For this review, take the finished solid that the model builds, in its own axes (mm). A direction names the side the tool comes from. Round coordinates to 2 decimals unless told otherwise and drop trailing zeros. Order: outer loops, then holes, each group sorted by start corner. A loop starts at its lowest first (then second) coordinate and runs counter-clockwise, first axis right, second up. Notation, with made-up numbers: M 64.25,56.25 L 91.25,56.25 A22 ccw 91.25,62.25 Z; hole C 10,-1 d10. An arc over 180 degrees is marked long. Answer as a JSON object with one key per item and string values.
from build123d import *

# Parameters (mm, degrees)
SKETCH1_R           = 18.5
BOSS_EXTRUDE1_DEPTH = 22
SKETCH2_R           = 16.5
BOSS_EXTRUDE2_DEPTH = 22
SKETCH3_R           = 16.55
BOSS_EXTRUDE3_DEPTH = 1
SKETCH4_R           = 6.5
BOSS_EXTRUDE4_DEPTH = 6
SKETCH6_R           = 3
BOSS_EXTRUDE5_DEPTH = 15.5
CUT_EXTRUDE1_DEPTH  = 12
SKETCH8_R           = 1.5
CUT_EXTRUDE2_DEPTH  = 10


with BuildPart() as part:
    # Sketch1 → Boss-Extrude1 (new body)
    with BuildSketch(Plane(origin=(0, 0, 0), x_dir=(1, 0, 0), z_dir=(0, 1, 0))):
        with Locations(Location((0, 0, 0), (0, 0, 270))):
            Circle(SKETCH1_R)
    extrude(amount=BOSS_EXTRUDE1_DEPTH)

    # Sketch2 → Boss-Extrude2 (add)
    with BuildSketch(Plane.XZ):
        with Locations(Location((0, 0, 0), (0, 0, 270))):
            Circle(SKETCH2_R)
    extrude(amount=BOSS_EXTRUDE2_DEPTH)

    # Sketch3 → Boss-Extrude3 (add)
    with BuildSketch(Plane.XZ.offset(22)):
        with Locations(Location((0, 0, 0), (0, 0, 270))):
            Circle(SKETCH3_R)
    extrude(amount=BOSS_EXTRUDE3_DEPTH)

    # Sketch4 → Boss-Extrude4 (add)
    with BuildSketch(Plane(origin=(0, 22, 0), x_dir=(1, 0, 0), z_dir=(0, 1, 0))):
        with Locations(Location((0, 7, 0), (0, 0, 270))):
            Circle(SKETCH4_R)
    extrude(amount=BOSS_EXTRUDE4_DEPTH)

    # Sketch6 → Boss-Extrude5 (add)
    with BuildSketch(Plane(origin=(0, 28, 0), x_dir=(1, 0, 0), z_dir=(0, 1, 0))):
        with Locations(Location((0, 7, 0), (0, 0, 270))):
            Circle(SKETCH6_R)
    extrude(amount=BOSS_EXTRUDE5_DEPTH)

    # Sketch7 → Cut-Extrude1 (cut)
    with BuildSketch(Plane(origin=(0, 43.5, 0), x_dir=(1, 0, 0), z_dir=(0, 1, 0))):
        Polygon((-2.084617871, 9.15739851), (2.084617871, 9.15739851), (2.280696351, 9.15739851), (2.280696351, 10.992904137), (-3.0808507, 10.992904137), (-3.0808507, 9.15739851), align=None)
    extrude(amount=-CUT_EXTRUDE1_DEPTH, mode=Mode.SUBTRACT)

    # Sketch8 → Cut-Extrude2 (cut)
    with BuildSketch(Plane(origin=(0, 22, 0), x_dir=(1, 0, 0), z_dir=(0, 1, 0))):
        with Locations(Location((15.5, 0, 0), (0, 0, 270))):
            Circle(SKETCH8_R)
        with Locations(Location((7.75, -13.423393759, 0), (0, 0, 270))):
            Circle(SKETCH8_R)
        with Locations(Location((-7.75, -13.423393759, 0), (0, 0, 270))):
            Circle(SKETCH8_R)
        with Locations(Location((-15.5, 0, 0), (0, 0, 270))):
            Circle(SKETCH8_R)
        with Locations(Location((-7.75, 13.423393759, 0), (0, 0, 270))):
            Circle(SKETCH8_R)
        with Locations(Location((7.75, 13.423393759, 0), (0, 0, 270))):
            Circle(SKETCH8_R)
    extrude(amount=-CUT_EXTRUDE2_DEPTH, mode=Mode.SUBTRACT)


solid = part.part
1) Insertion check: P1, Ø2.5, axis at x = -15.5, z = 0, coming from the +Y side; P2, Ø1, axis at x = -8.5, z = 4, coming from the +Y side; P3, Ø6, axis at x = -5.5, y = -5, coming from the +Z side. Each pin has a flat end and moves straight along its axis. Give the tip position at first contact, or say it passes through.
Geometry check:
{"P1": "stops at y = 12", "P2": "stops at y = 22", "P3": "stops at z = 16.31"}
2) Add section A-A on x = 0. State the section outline as (y, z) points.
Geometry check:
{"outline": "M -23,-16.55 L -22,-16.55 L -22,-16.5 L 0,-16.5 L 0,-18.5 L 22,-18.5 L 22,-13.5 L 28,-13.5 L 28,-10 L 31.5,-10 L 31.5,-9.16 L 43.5,-9.16 L 43.5,-4 L 28,-4 L 28,-0.5 L 22,-0.5 L 22,18.5 L 0,18.5 L 0,16.5 L -22,16.5 L -22,16.55 L -23,16.55 Z"}
3) Machinability: for faces 1 (the flat face through (0, 38, -9.157)), 2 (the cylindrical face through (6.84, 17.07, 12.23)), 3 (the cylindrical face through (4.971, -22.493, -15.786)), 4 (the cylindrical face through (-7.086, 10.846, 17.089)), which of the approach directions +Z, -Z, +X, -X, +Y, -Y give a long, thin tool a straight path to every point of the face, cutting with its end or side? Answer none if there is none.
Geometry check:
{"face 1": "-Z, +X, -X, +Y", "face 2": "+Y", "face 3": "-Y", "face 4": "+Y, -Y"}
4) Add section B-B on z = -7. State the section outline as (x, y) points.
Geometry check:
{"outline": "M -17.12,0 L -14.94,0 L -14.94,-22 L -15,-22 L -15,-23 L 15,-23 L 15,-22 L 14.94,-22 L 14.94,0 L 17.12,0 L 17.12,22 L 6.5,22 L 6.5,28 L 3,28 L 3,43.5 L -3,43.5 L -3,28 L -6.5,28 L -6.5,22 L -17.12,22 Z"}
5) Add section D-D on x = -13. State the section outline as (y, z) points, and give its area (3 significant figures).
Geometry check:
{"outline": "M -23,-10.24 L -22,-10.24 L -22,-10.16 L 0,-10.16 L 0,-13.16 L 22,-13.16 L 22,13.16 L 0,13.16 L 0,10.16 L -22,10.16 L -22,10.24 L -23,10.24 Z", "area": "1,050 mm²"}
6) Mouldability with a two-part tool opening along Z and no side actions: class faces 5 (the flat face through (0, 22, 0)), 6 (the cylindrical face through (-15.05, 17.07, 1.43)), 7 (the cylindrical face through (0.9, 35.64, -4.14)) as +Z half, -Z half, draft (parallel to the pull), parting line (faces both ways), or undercut.
Geometry check:
{"face 5": "draft", "face 6": "undercut", "face 7": "parting line"}
7) For L1, parallel to Z at x = 7, y = 17; L2, parallel to X at y = 16, z = 0; L3, parallel to Y at x = -5, z = -13, list the stretches that pass through material, from the lowest coordinate up.
Geometry check:
{"L1": "z = -17.12 to -14.72, -12.12 to 12.12, 14.72 to 17.12", "L2": "x = -18.5 to -17, -14 to 14, 17 to 18.5", "L3": "y = -23 to 22"}
8) Add section C-C on y = -8. State the section outline as (x, z) points, and give its area (3 significant figures).
Geometry check:
{"outline": "C 0,0 d33", "area": "855 mm²"}
